For this review, use the dimensioned drawing (mm, ordinates from the lowest corner) and the shaded views. Round coordinates to 2 decimals unless told otherwise and drop trailing zeros. Write each loop counter-clockwise with the first axis right and the second up, starting at its lowest first coordinate (ties: lowest second). Pieces come first, ordered by that corner, then holes. Notation, with made-up numbers: M 10,71 L 21,71 A25 cw 21,90 Z; hole C 63,-2 d7. An arc over 180 degrees is marked long. Use CSV: the item, a comma, the result in double quotes.
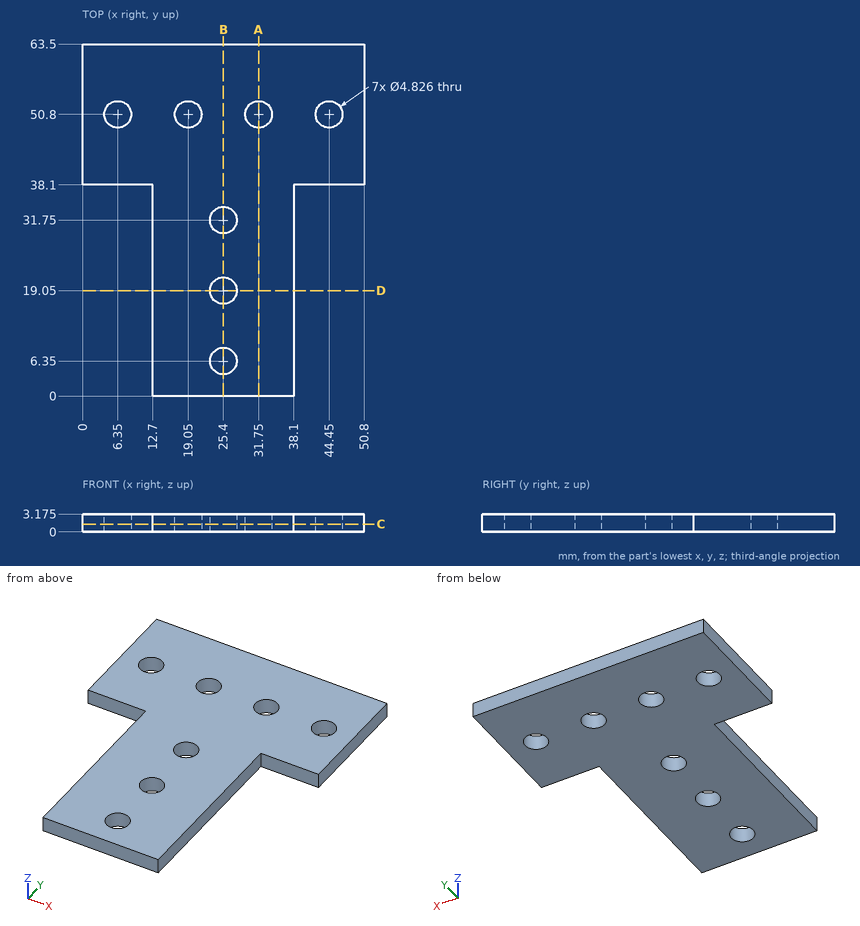
1) Add section D-D on y = 19.05. Write out the cut boundary in (x, z) (3 decimals), then the cut area to 3 significant figures.
Answers:
outline,"M 12.7,0 L 22.987,0 L 22.987,3.175 L 12.7,3.175 Z; M 27.813,0 L 38.1,0 L 38.1,3.175 L 27.813,3.175 Z"
area,"65.3 mm²"
2) Wall thickness on line 1 along Y through (x, z) = (25.4, 2.55); line 2 along Y through (x, z) = (19.05, 1); line 3 along X through (y, z) = (19, 0.6): over which ranges is each line inside the solid? List them lowest first. Write a range as [from, to].
Answers:
line 1,"[0, 3.94], [8.76, 16.64], [21.46, 29.34], [34.16, 63.5]"
line 2,"[0, 48.39], [53.21, 63.5]"
line 3,"[12.7, 22.99], [27.81, 38.1]"
3) Add section C-C on z = 1.4. Write out the cut boundary in (x, y), then the cut area to 3 significant figures.
Answers:
outline,"M 0,38.1 L 12.7,38.1 L 12.7,0 L 38.1,0 L 38.1,38.1 L 50.8,38.1 L 50.8,63.5 L 0,63.5 Z; hole C 6.35,50.8 d4.83; hole C 19.05,50.8 d4.83; hole C 25.4,6.35 d4.83; hole C 25.4,19.05 d4.83; hole C 25.4,31.75 d4.83; hole C 31.75,50.8 d4.83; hole C 44.45,50.8 d4.83"
area,"2,130 mm²"
4) Add section B-B on x = 25.4. Write out the cut boundary in (y, z) (3 decimals), then the cut area to 3 significant figures.
Answers:
outline,"M 0,0 L 3.937,0 L 3.937,3.175 L 0,3.175 Z; M 8.763,0 L 16.637,0 L 16.637,3.175 L 8.763,3.175 Z; M 21.463,0 L 29.337,0 L 29.337,3.175 L 21.463,3.175 Z; M 34.163,0 L 63.5,0 L 63.5,3.175 L 34.163,3.175 Z"
area,"156 mm²"
5) Add section A-A on x = 31.75. Write out the cut boundary in (y, z) (3 decimals), then the cut area to 3 significant figures.
Answers:
outline,"M 0,0 L 48.387,0 L 48.387,3.175 L 0,3.175 Z; M 53.213,0 L 63.5,0 L 63.5,3.175 L 53.213,3.175 Z"
area,"186 mm²"
6) For pin 1 Ø1.6 at (x, z) = (5.5, 1.5) entering from -Y; pin 2 Ø5.5 at (x, y) = (25.4, 31.75) entering from +Z (3 decimals), all flat-tipped, find the tip position at first contact; note any pin that passes through.
Answers:
pin 1,"y = 38.1"
pin 2,"z = 3.175"
